Source: CAD feature listing. Evaluate the final solid. Frame: model axes, mm. Give positions to 0.01 mm unless a question says otherwise; leave off trailing zeros. Loops run counter-clockwise (first coordinate to the right, second up) from the corner with the lowest first, then second, coordinate; pieces in that order, holes last. Notation, with made-up numbers: M 35,3 L 53,3 A20 cw 53,28 Z; hole C 77.25,-29.5 d7. An arc over 180 degrees is marked long. Answer in a Markdown table with one row per item.
Autodesk Fusion 360 part; units mm, degrees
sketch "Sketch1" plane through (0, 0, 0) normal (0, 0, 1) x (1, 0, 0)
  circle A0 centre (0, 0) radius 25
  line L0 (-250, 100) -> (250, 100)
  line L1 (250, 100) -> (250, -100)
  line L2 (250, -100) -> (-250, -100)
  line L3 (-250, -100) -> (-250, 100)
  line L4 (-250, 0) -> (250, 0) construction
  line L5 (0, 100) -> (0, -100) construction
  dimension "Total_Width" = 500
  dimension "Total_Height" = 200
  dimension "Hole_Radius" = 25
extrude "Extrude1" add sketch "Sketch1" along normal mid plane 10
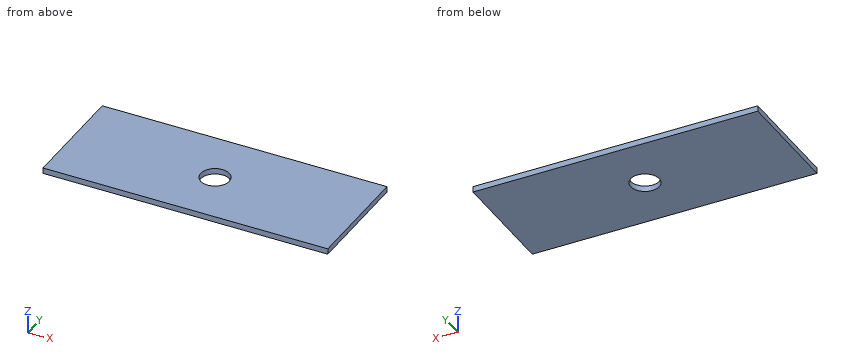
1) Material intervals for L1, parallel to Y at x = 0, z = -0.75; L2, parallel to X at y = 19, z = -2.25; L3, parallel to X at y = -5, z = -1, sorted ascending.
Reply:
| item | result |
|---|---|
| L1 | y = -100 to -25, 25 to 100 |
| L2 | x = -250 to -16.25, 16.25 to 250 |
| L3 | x = -250 to -24.49, 24.49 to 250 |
2) Section C-C, the plane z = 2.5. Return loops of the section in (x, y).
Reply:
| item | result |
|---|---|
| outline | M -250,-100 L 250,-100 L 250,100 L -250,100 Z; hole C 0,0 d50 |
3) Section A-A, the plane y = 0. Return loops of the section in (x, z), then the cut area to 3 significant figures.
Reply:
| item | result |
|---|---|
| outline | M -250,-5 L -25,-5 L -25,5 L -250,5 Z; M 25,-5 L 250,-5 L 250,5 L 25,5 Z |
| area | 4,500 mm² |
4) Section B-B, the plane x = 0. Return loops of the section in (y, z), then the cut area to 3 significant figures.
Reply:
| item | result |
|---|---|
| outline | M -100,-5 L -25,-5 L -25,5 L -100,5 Z; M 25,-5 L 100,-5 L 100,5 L 25,5 Z |
| area | 1,500 mm² |
